```python
from build123d import *

# Parameters (mm, degrees)
F2_R = 10.0418427949
F3_R = 5
F4_R = 5
F5_R = 5
F6_R = 5
F7_R = 5
F8_R = 5
F9_R = 5


with BuildPart() as f1:
    # F0 (on Top) → F1 (revolve)
    with BuildSketch(Plane.XY):
        with BuildLine():
            Line((3.9978994305, 41.8078787625), (0, 45.2654622495))
            Line((0, 45.2654622495), (0, -46.6173030436))
            add(Edge.make_bspline(
                [(19.1201921552, -40.0373525918), (17.3987358712, -41.8425355299), (13.410823789, -46.0244081204), (4.8598099626, -46.4024499742), (0, -46.6173030436)],
                knots=[0, 0, 0, 0, 0.4316685645, 1, 1, 1, 1], degree=3))
            Line((19.1201921552, -40.0373525918), (19.1201921552, -33.4124453366))
            Line((19.1201921552, -33.4124453366), (16.8782249093, -12.2566334903))
            Line((16.8782249093, -12.2566334903), (19.1201921552, -10.3883286938))
            Line((19.1201921552, -10.3883286938), (19.1201921552, -5.157073494))
            Line((19.1201921552, -5.157073494), (16.8782249093, 1.5688246349))
            Line((16.8782249093, 1.5688246349), (19.1201921552, 3.4371297807))
            Line((19.1201921552, 3.4371297807), (19.1201921552, 10.910349898))
            Line((19.1201921552, 10.910349898), (19.1201921552, 13.8996383175))
            Line((19.1201921552, 13.8996383175), (16.8782249093, 20.2518757433))
            Line((16.8782249093, 20.2518757433), (11.4163085818, 20.2518757433))
            Line((11.4163085818, 20.2518757433), (11.4163085818, 22.2149007022))
            Line((11.4163085818, 22.2149007022), (11.4163085818, 27.1131433547))
            Line((11.4163085818, 27.1131433547), (3.9978994305, 33.7401814759))
            Line((3.9978994305, 33.7401814759), (3.9978994305, 41.8078787625))
        make_face()
    revolve(axis=Axis((0, -0.675920397, 0), (0, -1, 0)))

    # F2
    f2_edges = [f1.edges().sort_by_distance(p)[0] for p in [
        (-3.997899, 41.807879, 0),
        (1.99895, 43.536671, 0),
    ]]
    fillet(f2_edges, radius=F2_R)

    # F3
    f3_edges = [f1.edges().sort_by_distance(p)[0] for p in [
        (-16.878225, 20.251876, 0),
    ]]
    fillet(f3_edges, radius=F3_R)

    # F4
    f4_edges = [f1.edges().sort_by_distance(p)[0] for p in [
        (-19.120192, -5.157073, 0),
    ]]
    fillet(f4_edges, radius=F4_R)

    # F5
    f5_edges = [f1.edges().sort_by_distance(p)[0] for p in [
        (-11.416309, 27.113143, 0),
    ]]
    fillet(f5_edges, radius=F5_R)

    # F6
    f6_edges = [f1.edges().sort_by_distance(p)[0] for p in [
        (-11.416309, 20.251876, 0),
    ]]
    fillet(f6_edges, radius=F6_R)

    # F7
    f7_edges = [f1.edges().sort_by_distance(p)[0] for p in [
        (-19.120192, -10.388329, 0),
    ]]
    fillet(f7_edges, radius=F7_R)

    # F8
    f8_edges = [f1.edges().sort_by_distance(p)[0] for p in [
        (-16.878225, -12.256633, 0),
    ]]
    fillet(f8_edges, radius=F8_R)

    # F9
    f9_edges = [f1.edges().sort_by_distance(p)[0] for p in [
        (-19.120192, 3.43713, 0),
    ]]
    fillet(f9_edges, radius=F9_R)


solid = f1.part
```
Input: part model. Units: mm. Frame: model coordinates. A direction names the side the tool comes from. Coordinates: 2 decimals unless noted, no trailing zeros. Loops run counter-clockwise (first coordinate to the right, second up) from the corner with the lowest first, then second, coordinate; pieces in that order, holes last. Notation, with made-up numbers: (-33, -8) - (8, -8) arc R16 cw to (8, 2) - close; hole circle Ø3 at (32, 19). An arc over 180 degrees is marked (long way). Answer in a Markdown table with one row per item.
(1) Set-up query: faces 4 (the face through (3.693, 35.503, -1.531)), 5 (the face through (17.662, 9.896, -7.323)), 6 (the face through (-3.68, 1.28, -16.57)). Return all of +Z, -Z, +X, -X, +Y, -Y with unobstructed straight access to the full face (end or side cutting, diameter ignored); none if empty.
Model answer:
| item | result |
|---|---|
| face 4 | +Y |
| face 5 | +Y, -Y |
| face 6 | none |
(2) Mould query, pull axis Y, two halves, no side actions, for faces 1 (the face through (-0.927, 33.491, -4.175)), 2 (the face through (8.823, -36.679, -16.963)), 3 (the face through (17.062, -21.785, 5.373)). Classes: pulls with the +Y half, pulls with the -Y half, needs draft (parallel to the pull), parting line crosses it, or undercut.
Model answer:
| item | result |
|---|---|
| face 1 | pulls with the +Y half |
| face 2 | needs draft |
| face 3 | undercut |
(3) Material intervals for L1, parallel to Z at x = 1, y = -11; L2, parallel to Z at x = -7.5, y = 26.5; L3, parallel to X at y = -37, z = 0.5, sorted ascending. Write a range as from..to.
Model answer:
| item | result |
|---|---|
| L1 | z = -18.13..18.13 |
| L2 | z = -8.24..8.24 |
| L3 | x = -19.11..19.11 |
(4) Cut plane A-A on y = -17. Output: boundary loops of the cut face in (x, z), plus the area to 3 significant figures.
Model answer:
| item | result |
|---|---|
| outline | circle Ø34.76 at (0, 0) |
| area | 949 mm² |
(5) Pin query (flat end, axial travel): P1, Ø12, axis at x = 12, z = -12, coming from the +Y side; P2, Ø1, axis at x = 15, z = -10, coming from the -Y side; P3, Ø8, axis at x = -14, y = 24.5, coming from the +Z side. Return the tip coordinate at first contact, or that it passes through.
Model answer:
| item | result |
|---|---|
| P1 | stops at y = 26.94 |
| P2 | stops at y = -41.66 |
| P3 | stops at z = 5.66 |
